Source: CAD feature listing. Evaluate the final solid. Frame: model axes, mm. Face numbers are marked on the shaded views. Give positions to 0.01 mm unless a question says otherwise; leave off trailing zeros. Loops run counter-clockwise (first coordinate to the right, second up) from the corner with the lowest first, then second, coordinate; pieces in that order, holes last.
from build123d import *

# Parameters (mm, degrees)
F1_DEPTH = 2
F2_R     = 3.25
F3_DEPTH = 9
F5_D     = 3
F5_DEPTH = 9
F5_TIP   = 0.9012909285


with BuildPart() as f1:
    # F0 (on Top) → F1 (new body)
    with BuildSketch(Plane.XY):
        with BuildLine():
            ThreePointArc((21, 17.35), (19.5355339059, 20.8855339059), (16, 22.35))
            Line((16, 22.35), (-16, 22.35))
            ThreePointArc((-16, 22.35), (-19.5355339059, 20.8855339059), (-21, 17.35))
            Line((-21, 17.35), (-21, -17.35))
            ThreePointArc((-21, -17.35), (-19.5355339059, -20.8855339059), (-16, -22.35))
            Line((-16, -22.35), (16, -22.35))
            ThreePointArc((16, -22.35), (19.5355339059, -20.8855339059), (21, -17.35))
            Line((21, -17.35), (21, 17.35))
        make_face()
    extrude(amount=F1_DEPTH)

    # F2 (on face) → F3 (join)
    with BuildSketch(Plane.XY.offset(2)):
        with Locations((13.5, -14.75)):
            Circle(F2_R)
        with Locations((-13.5, 14.75)):
            Circle(F2_R)
        with Locations((13.5, 14.75)):
            Circle(F2_R)
        with Locations((-13.5, -14.75)):
            Circle(F2_R)
    extrude(amount=F3_DEPTH)

    # F5
    with Locations(Plane.XY.offset(11)):
        with Locations((-13.5, 14.75), (13.5, 14.75), (13.5, -14.75), (-13.5, -14.75)):
            Hole(F5_D / 2, depth=F5_DEPTH)
            with Locations((0, 0, -(F5_DEPTH + F5_TIP / 2))):  # 118° drill point
                Cone(0, F5_D / 2, F5_TIP, mode=Mode.SUBTRACT)


solid = f1.part
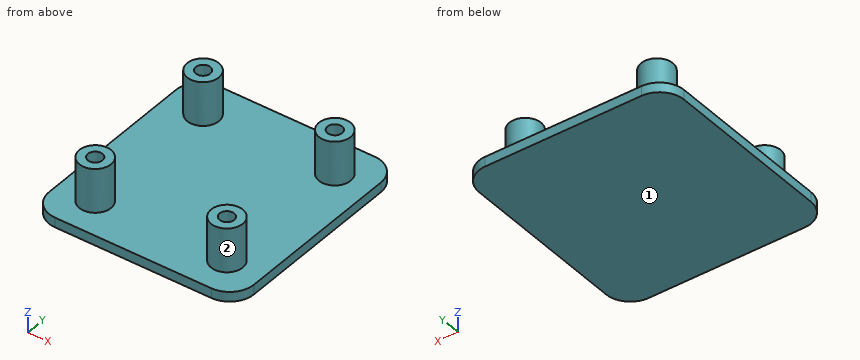
1) Cut plane A-A (z = 8.5). Return loops of the section in (x, y).
Checks:
outline: circle Ø6.5 at (-13.5, -14.75); circle Ø6.5 at (-13.5, 14.75); circle Ø6.5 at (13.5, -14.75); circle Ø6.5 at (13.5, 14.75); hole circle Ø3 at (-13.5, -14.75); hole circle Ø3 at (-13.5, 14.75); hole circle Ø3 at (13.5, -14.75); hole circle Ø3 at (13.5, 14.75)
2) Cut plane B-B (x = 7). Return loops of the section in (y, z), and give its area (3 significant figures).
Checks:
outline: (-22.35, 0) - (22.35, 0) - (22.35, 2) - (-22.35, 2) - close
area: 89.4 mm2
3) Contact query for flat-ended pins moving along their axis: P1, Ø4, axis at y = 12, z = 5.5, coming from the +X side; P2, Ø10, axis at x = 1.5, y = -9.5, coming from the +Z side; P3, Ø2.5, axis at x = 13.5, y = 14.75, coming from the +Z side. Output: stop coordinate, or through.
Checks:
P1: stops at x = 16.66
P2: stops at z = 2
P3: stops at z = 1.85
4) Pull-direction query (X, two-part tool) for the marked faces 1 and 2; classes: released by +X, released by -X, zero draft, split by the parting line, or undercut.
Checks:
face 1: zero draft
face 2: undercut
5) Cut plane C-C (y = 11). Return loops of the section in (x, z).
Checks:
outline: (-21, 0) - (21, 0) - (21, 2) - (-21, 2) - close
6) Ray query, probe 1 along Y at (x, z) = (13.5, 7.5); probe 2 along Y at (x, z) = (14.5, 6.75); probe 3 along X at (y, z) = (-16, 6.75). Return the intervals inside material, ascending.
Checks:
probe 1: y = -18 to -16.25, -13.25 to -11.5, 11.5 to 13.25, 16.25 to 18
probe 2: y = -17.84 to -15.87, -13.63 to -11.66, 11.66 to 13.63, 15.87 to 17.84
probe 3: x = -16.5 to -14.33, -12.67 to -10.5, 10.5 to 12.67, 14.33 to 16.5
